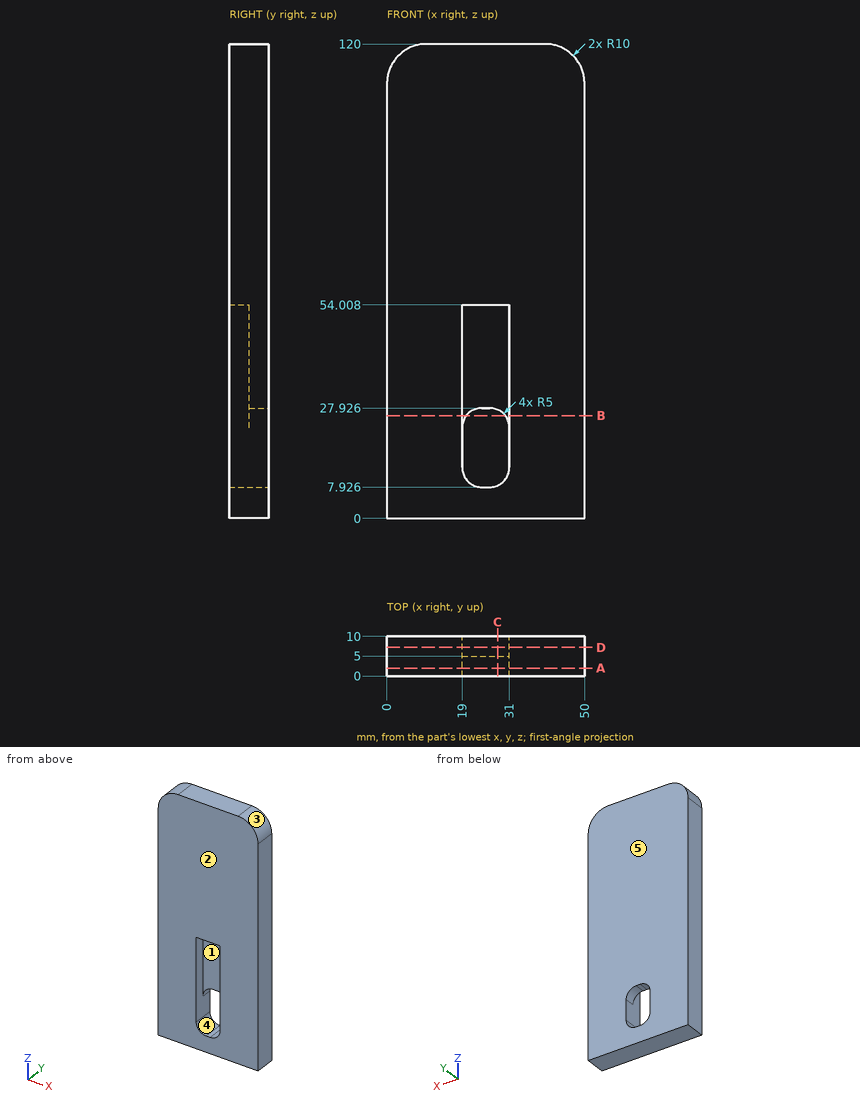
Job drawing, mm, ordinate dimensions from the low corner. One solid piece. A direction names the side the tool comes from. Coordinates: 2 decimals unless noted, no trailing zeros. Write each loop counter-clockwise with the first axis right and the second up, starting at its lowest first coordinate (ties: lowest second). Pieces come first, ordered by that corner, then holes.
Item 1: Slice it at C-C (x = 28). Write the cut outline in (y, z).
Item 2: Mould opens along Z. For the marked faces 1, 2 and 3 say: released by +Z, released by -Z, zero draft, split by the parting line, or undercut.
Item 3: Slice it at D-D (y = 7.25). Write the cut outline in (x, z) (1 decimal), and give its area (3 significant figures).
Item 4: Probe line 1 (Z direction, x = 23.5, y = 2.25); line 2 (X direction, y = 3.5, z = 29); line 3 (Z direction, x = 25, y = 2.75) (1 decimal). List the from-to ranges inside material, lowest first.
Item 5: Slice it at A-A (y = 2). Write the cut outline in (x, z) (1 decimal).
Item 6: Which spindle directions (+Z, -Z, +X, -X, +Y, -Y) get a long thin tool onto all of the face, cutting with end or side? Do the marked faces 4 and 5. Say none if no direction does.
Item 7: Slice it at B-B (z = 26). Write the cut outline in (x, y).
Results found:
1. outline: (0, 0) - (10, 0) - (10, 8.34) - (0, 8.34) - close; (0, 54.01) - (5, 54.01) - (5, 27.51) - (10, 27.51) - (10, 120) - (0, 120) - close
2. face 1: undercut
2. face 2: zero draft
2. face 3: released by +Z
3. outline: (0, 0) - (50, 0) - (50, 110) arc R10 ccw to (40, 120) - (10, 120) arc R10 ccw to (0, 110) - close; hole (19, 12.9) arc R5 ccw to (24, 7.9) - (26, 7.9) arc R5 ccw to (31, 12.9) - (31, 22.9) arc R5 ccw to (26, 27.9) - (24, 27.9) arc R5 ccw to (19, 22.9) - close
3. area: 5,740 mm2
4. line 1: z = 0 to 7.95, 54.01 to 120
4. line 2: x = 0 to 19, 31 to 50
4. line 3: z = 0 to 7.9, 54 to 120
5. outline: (0, 0) - (50, 0) - (50, 110) arc R10 ccw to (40, 120) - (10, 120) arc R10 ccw to (0, 110) - close; hole (19, 12.9) arc R5 ccw to (24, 7.9) - (26, 7.9) arc R5 ccw to (31, 12.9) - (31, 54) - (19, 54) - close
6. face 4: +Y, -Y
6. face 5: +Z, -Z, +X, -X, +Y
7. outline: (0, 0) - (19, 0) - (19, 5) - (20.06, 5) - (20.06, 10) - (0, 10) - close; (29.94, 5) - (31, 5) - (31, 0) - (50, 0) - (50, 10) - (29.94, 10) - close
